Design review of the part built by this model. Coordinates are the model's own, in mm. A direction names the side the tool comes from. Round coordinates to 2 decimals unless told otherwise and drop trailing zeros. Loops run counter-clockwise (first coordinate to the right, second up) from the corner with the lowest first, then second, coordinate; pieces in that order, holes last. Notation, with made-up numbers: (-21.5, -3) - (-0.5, -3) arc R25 ccw to (-0.5, 13) - close; hole circle Ø11 at (-21.75, -26). An arc over 180 degrees is marked (long way). Return JSON: item names as keys, results as strings. Group by question number.
Autodesk Fusion 360 part; units mm, degrees
sketch "Sketch1" plane through (0, 0, 0) normal (0, 1, 0) x (1, 0, 0)
  line L0 (0, 0) -> (-70, 0)
  line L1 (-70, 0) -> (-70, 70)
  line L2 (-70, 70) -> (0, 70)
  line L3 (0, 70) -> (0, 0)
  dimension "d1" = 70
  dimension "d2" = 70
extrude "Extrude1" add sketch "Sketch1" along normal blind 2
sketch "Sketch2" plane through (0, 2, 0) normal (0, 1, 0) x (-1, 0, 0)
  line L0 (0, -70) -> (70, -70)
  line L1 (70, -70) -> (70, 0)
  line L2 (70, 0) -> (0, 0)
  line L3 (0, 0) -> (0, -70)
  line L4 (62.0012, -62.7393) -> (32.0012, -62.7393)
  line L5 (32.0012, -62.7393) -> (32.0012, -41.2393)
  line L6 (32.0012, -41.2393) -> (62.0012, -41.2393)
  line L7 (62.0012, -41.2393) -> (62.0012, -62.7393)
  line L8 (13.8147, -60) -> (11, -60)
  line L9 (25, -45) -> (25, -47.8147)
  line L10 (62.0012, -62.7393) -> (63.4154, -62.7393) construction
  line L11 (32.0012, -41.2393) -> (33.4154, -41.2393) construction
  line L12 (63.0012, -63.7393) -> (31.0012, -63.7393)
  line L13 (31.0012, -63.7393) -> (31.0012, -40.2393)
  line L14 (31.0012, -40.2393) -> (63.0012, -40.2393)
  line L15 (63.0012, -40.2393) -> (63.0012, -63.7393)
  line L16 (13.8147, -61) -> (9.8147, -61)
  line L17 (26, -43.8147) -> (26, -47.8147)
  line L18 (62.0012, -62.7393) -> (66.2472, -62.7393) construction
  circle A0 centre (58.9988, -59.7369) radius 1
  line L19 (26, -61) -> (22, -61)
  line L20 (9.8147, -61) -> (13.8147, -61)
  line L21 (13.8147, -61) -> (13.8147, -60)
  line L22 (9.8147, -61) -> (9.8147, -57.5477)
  line L23 (9.8147, -57.5477) -> (11, -57.5477)
  line L24 (9.8147, -43.8147) -> (9.8147, -47.8147)
  line L25 (11, -47.8147) -> (9.8147, -47.8147)
  line L26 (9.8147, -43.8147) -> (13.8147, -43.8147)
  line L27 (13.8147, -45) -> (13.8147, -43.8147)
  line L28 (26, -43.8147) -> (22, -43.8147)
  line L29 (22, -43.8147) -> (22, -45)
  line L30 (26, -43.8147) -> (26, -47.8147)
  line L31 (25, -47.8147) -> (26.1763, -47.8147)
  line L32 (11, -45) -> (13.8147, -45)
  line L33 (22, -45) -> (25, -45)
  line L34 (9.8147, -43.8147) -> (13.8147, -43.8147)
  line L35 (22, -43.8147) -> (26, -43.8147)
  line L36 (26, -61) -> (26, -57)
  line L37 (26, -57) -> (25, -57)
  line L38 (25, -57) -> (25, -60)
  line L39 (22, -61) -> (22, -60)
  line L40 (22, -60) -> (25, -60)
  line L41 (9.8147, -61) -> (9.8147, -57.5477)
  line L42 (9.8147, -47.8147) -> (9.8147, -43.8147)
  line L43 (11, -60) -> (11, -57.5477)
  line L44 (11, -47.8147) -> (11, -45)
  line L45 (33.8182, -10.0332) -> (4.8182, -10.0332)
  line L46 (58.5866, -26.0332) -> (4.8182, -26.0332)
  line L47 (33.8182, -9.5332) -> (4.3182, -9.5332)
  line L48 (4.8182, -10.0332) -> (62.8182, -10.0332)
  line L49 (63.3182, -26.5332) -> (4.3182, -26.5332)
  line L50 (4.8182, -16.9457) -> (4.8182, -10.0332)
  line L51 (4.3182, -26.5332) -> (4.3182, -9.5332)
  line L52 (58.5866, -26.0332) -> (62.8182, -26.0332)
  line L53 (63.3182, -9.5332) -> (63.3182, -26.5332)
  line L54 (4.8182, -16.9457) -> (4.8182, -26.0332)
  line L55 (33.8182, -9.5332) -> (63.3182, -9.5332)
  line L56 (62.8182, -19.4958) -> (62.8182, -10.0332)
  line L57 (33.8182, -10.0332) -> (62.8182, -10.0332)
  line L58 (62.8182, -19.4958) -> (62.8182, -26.0332)
  line L59 (33.8182, -10.0332) -> (33.8182, -9.5332)
  line L60 (31.0012, -40.2393) -> (36.6612, -40.2393) construction
  circle A1 centre (35.0034, -44.2415) radius 1
  line L61 (63.0012, -40.2393) -> (68.6612, -40.2393) construction
  line L62 (31.0012, -63.7393) -> (36.6612, -63.7393) construction
  circle A2 centre (35.0034, -59.7371) radius 1
  circle A3 centre (58.9989, -44.2415) radius 1
  point P0 (33.8182, -10.0332)
  dimension "d5" = 30
  dimension "d6" = 21.5
  dimension "d7" = 14
  dimension "d8" = 15
  dimension "d9" = 1.4142
  dimension "d12" = 1.4142
  dimension "d14" = 4.246
  dimension "d15" = 2
  dimension "d34" = 4
  dimension "d35" = 4
  dimension "d36" = 4
  dimension "d37" = 4
  dimension "d38" = 4
  dimension "d39" = 4
  dimension "d72" = 0.5
  dimension "d76" = 5.66
  dimension "d77" = 2
  dimension "d79" = 5.66
  dimension "d80" = 5.66
  dimension "d82" = 2
  dimension "d83" = 2
extrude "Extrude2" add sketch "Sketch2" along normal blind 4 contours A0
extrude "Extrude7" add sketch "Sketch2" along normal blind 4 contours A1 | A2 | A3
extrude "Extrude3" add sketch "Sketch2" along normal blind 1.5 contours L12 L13 L14 L15
extrude "Extrude4" add sketch "Sketch2" along normal blind 1.5 contours L8 L16 L20 L21 L22 L23 L41 L43 | L9 L17 L28 L29 L30 L31 L33 L35 | L19 L36 L37 L38 L39 L40 | L24 L25 L26 L27 L32 L34 L42 L44
sketch "Sketch3" plane through (0, 2, 0) normal (0, 1, 0) x (-1, 0, 0)
  line L0 (70, -70) -> (74, -70) construction
  line L1 (0, 0) -> (4, 0) construction
  line L2 (64.5858, -68.5858) -> (5.4142, -68.5858)
  line L3 (1.4142, -64.5858) -> (1.4142, -5.4142)
  line L4 (5.4142, -1.4142) -> (64.5858, -1.4142)
  line L5 (68.5858, -5.4142) -> (68.5858, -64.5858)
  line L6 (5.4142, -1.4142) -> (5.4142, -5.4142)
  line L7 (1.4142, -5.5403) -> (1.4142, -5.4142)
  line L8 (5.4142, -1.4142) -> (5.4142, -5.4142)
  line L9 (5.4142, -5.4142) -> (1.4142, -5.4142)
  line L10 (64.5858, -1.4142) -> (64.5858, -5.4142)
  line L11 (64.5858, -5.4142) -> (68.5858, -5.4142)
  line L12 (64.5858, -68.5858) -> (64.5858, -64.5858)
  line L13 (64.5858, -64.5858) -> (68.5858, -64.5858)
  line L14 (5.4142, -68.5858) -> (5.4142, -64.5858)
  line L15 (5.4142, -64.5858) -> (1.4142, -64.5858)
  line L16 (0, 0) -> (70, 0)
  line L17 (70, 0) -> (70, -70)
  line L18 (70, -70) -> (0, -70)
  line L19 (0, -70) -> (0, 0)
extrude "Extrude5" add sketch "Sketch3" along normal blind 15
hole "Hole1" at (-1.4142, 9.0391, -48.9799) direction (1, 0, 0) diameter 1 depth 14 tip angle 180
hole "Hole2" at (-1.4142, 8.6563, -26.0128) direction (1, 0, 0) diameter 1 depth 14 tip angle 180
hole "Hole3" at (-19.7207, 8.7497, -1.4142) direction (0, 0, 1) diameter 1 depth 14 tip angle 180
hole "Hole4" at (-44.3914, 9.679, -1.4142) direction (0, 0, 1) diameter 1 depth 14 tip angle 180
hole "Hole5" at (-68.5858, 9.867, -41.5184) direction (-1, 0, 0) diameter 1 depth 14 tip angle 180
hole "Hole6" at (-68.5858, 9.5121, -25.466) direction (-1, 0, 0) diameter 1 depth 14 tip angle 180
hole "Hole7" at (-44.6422, 9.2674, -68.5858) direction (0, 0, -1) diameter 1 depth 14 tip angle 180
hole "Hole8" at (-28.6065, 9.472, -68.5858) direction (0, 0, -1) diameter 1 depth 14 tip angle 180
sketch "Sketch4" plane through (0, 17, 0) normal (0, 1, 0) x (-1, 0, 0)
  line L0 (64.5858, -64.5858) -> (64.5858, -68.5858)
  line L1 (64.5858, -68.5858) -> (5.4142, -68.5858)
  line L2 (5.4142, -68.5858) -> (5.4142, -64.5858)
  line L3 (5.4142, -64.5858) -> (1.4142, -64.5858)
  line L4 (1.4142, -64.5858) -> (1.4142, -5.4142)
  line L5 (1.4142, -5.4142) -> (5.4142, -5.4142)
  line L6 (5.4142, -5.4142) -> (5.4142, -1.4142)
  line L7 (5.4142, -1.4142) -> (64.5858, -1.4142)
  line L8 (64.5858, -1.4142) -> (64.5858, -5.4142)
  line L9 (64.5858, -5.4142) -> (68.5858, -5.4142)
  line L10 (68.5858, -5.4142) -> (68.5858, -64.5858)
  line L11 (68.5858, -64.5858) -> (64.5858, -64.5858)
  line L12 (0, -70) -> (70, -70)
  line L13 (70, -70) -> (70, 0)
  line L14 (70, 0) -> (0, 0)
  line L15 (0, 0) -> (0, -70)
  line L16 (70, 0) -> (67.2928, -2.7072)
  line L17 (0, 0) -> (2.7072, -2.7072)
  line L18 (0, -70) -> (2.7071, -67.2929)
  line L19 (70, -70) -> (67.2929, -67.2929)
  dimension "d67" = 3.8285
  dimension "d68" = 3.8285
hole "Hole9" at (-2.7072, 17, -2.7072) at (-67.2928, 17, -2.7072) at (-67.2929, 17, -67.2929) at (-2.7071, 17, -67.2929) direction (0, -1, 0) diameter 4 depth 14 tip angle 180
sketch "Sketch5" plane through (0, 2, 0) normal (0, 1, 0) x (-1, 0, 0)
extrude "Extrude6" add sketch "Sketch2" along normal blind 2 contours L47 L49 L51 L53 L55
fillet "Fillet1" radius 2 1 edges at (-64.5858, 9.5, -64.5858)
fillet "Fillet2" radius 2 3 edges at (-5.4142, 9.5, -5.4142) (-5.4142, 9.5, -64.5858) (-64.5858, 9.5, -5.4142)
fillet "Fillet3" radius 2 3 edges at (-70, 8.5, -70) (0, 8.5, -70) (-70, 8.5, 0)
fillet "Fillet4" radius 2 1 edges at (0, 8.5, 0)
equation "d9 = ( sqrt(2) ) * 1 mm"
equation "d12 = ( sqrt(2) ) * 1 mm"
equation "d67 = 7.657 mm / 2"
equation "d68 = 7.657 mm / 2"
Q1. For line 1 (Z direction, x = -46.5, y = 12); line 2 (Z direction, x = -3, y = 3.5), list the stretches that pass through material, from the lowest coordinate up.
Q2. Insertion check: pin 1 Ø1 at (x, z) = (-34.5, -31.5) entering from -Y; pin 2 Ø1.2 at (x, z) = (-68.5, -67) entering from +Y; pin 3 Ø3 at (x, z) = (-23, -45) entering from +Y; pin 4 Ø0.6 at (x, z) = (-58.5, -60) entering from +Y. Each pin has a flat end and moves straight along its axis. Give the tip position at first contact, or say it passes through.
Q3. Add section B-B, the plane x = -42. State the section outline as (y, z) points.
Q4. Add section A-A, the plane z = -30. State the section outline as (x, y) points, plus the area to 3 significant figures.
Q5. Tool access review of faces 4 (the cylindrical face through (-69.43, 8.38, -69.4)), 5 (the cylindrical face through (-4.844, 9.605, -65.187)): name each direction out of +Z, -Z, +X, -X, +Y, -Y from which nothing blocks a thin tool from reaching the whole face with its end or side.
Q6. Draft analysis for pull direction X (two halves, no side actions). For faces 1 (the flat face through (-59, 6, -60)), 2 (the flat face through (-35, 8, 0)), 3 (the cylindrical face through (-69.4, 8.38, -0.57)), state which applies: pulls with the +X half, pulls with the -X half, needs draft (parallel to the pull), parting line crosses it, or undercut.
Q7. Add section D-D, the plane z = -23. State the section outline as (x, y) points, plus the area to 3 significant figures.
Q8. Add section C-C, the plane y = 12.5. State the section outline as (x, z) points, plus the area to 3 significant figures.
Evaluation:
{
 "1": {"line 1": "-70 to -68.59, -1.41 to 0", "line 2": "-70 to -69.27, -65.31 to -64.59, -5.41 to -4.69, -0.73 to 0"},
 "2": {"pin 1": "y = 0", "pin 2": "y = 3", "pin 3": "y = 3.5", "pin 4": "y = 6"},
 "3": {"outline": "(0, -70) - (17, -70) - (17, -68.59) - (2, -68.59) - (2, -63.74) - (3.5, -63.74) - (3.5, -62.74) - (2, -62.74) - (2, -41.24) - (3.5, -41.24) - (3.5, -40.24) - (2, -40.24) - (2, -26.53) - (4, -26.53) - (4, -26.03) - (2, -26.03) - (2, -10.03) - (4, -10.03) - (4, -9.53) - (2, -9.53) - (2, -1.41) - (17, -1.41) - (17, 0) - (0, 0) - close"},
 "4": {"outline": "(-70, 0) - (0, 0) - (0, 17) - (-1.41, 17) - (-1.41, 2) - (-68.59, 2) - (-68.59, 17) - (-70, 17) - close", "area": "182 mm²"},
 "5": {"face 4": "-Z, -X, +Y, -Y", "face 5": "+Y"},
 "6": {"face 1": "undercut", "face 2": "needs draft", "face 3": "pulls with the -X half"},
 "7": {"outline": "(-70, 0) - (0, 0) - (0, 17) - (-1.41, 17) - (-1.41, 2) - (-4.32, 2) - (-4.32, 4) - (-4.82, 4) - (-4.82, 2) - (-62.82, 2) - (-62.82, 4) - (-63.32, 4) - (-63.32, 2) - (-68.59, 2) - (-68.59, 17) - (-70, 17) - close", "area": "184 mm²"},
 "8": {"outline": "(-70, -68) arc R2 ccw to (-68, -70) - (-2, -70) arc R2 ccw to (0, -68) - (0, -2) arc R2 ccw to (-2, 0) - (-68, 0) arc R2 ccw to (-70, -2) - close; hole circle Ø4 at (-67.29, -67.29); hole circle Ø4 at (-67.29, -2.71); hole (-68.59, -64.59) - (-66.59, -64.59) arc R2 cw to (-64.59, -66.59) - (-64.59, -68.59) - (-5.41, -68.59) - (-5.41, -66.59) arc R2 cw to (-3.41, -64.59) - (-1.41, -64.59) - (-1.41, -5.41) - (-3.41, -5.41) arc R2 cw to (-5.41, -3.41) - (-5.41, -1.41) - (-64.59, -1.41) - (-64.59, -3.41) arc R2 cw to (-66.59, -5.41) - (-68.59, -5.41) - close; hole circle Ø4 at (-2.71, -67.29); hole circle Ø4 at (-2.71, -2.71)", "area": "395 mm²"}
}
